Source: CAD feature listing. Evaluate the final solid. Frame: model axes, mm. A direction names the side the tool comes from. Coordinates: 2 decimals unless noted, no trailing zeros. Write each loop counter-clockwise with the first axis right and the second up, starting at its lowest first coordinate (ties: lowest second). Pieces come first, ordered by that corner, then holes. Notation, with made-up numbers: (61, 0) - (99, 0) arc R16 ccw to (99, 24) - close; hole circle Ø11 at (-11.5, -39.5). An arc over 180 degrees is marked (long way). One line per question, with ' | ' between items.
Autodesk Inventor part; units mm, degrees
ref_plane "YZ Plane" through (0, 0, 0) normal (1, 0, 0) x (0, 1, 0)
ref_plane "XZ Plane" through (0, 0, 0) normal (0, 1, 0) x (-1, 0, 0)
ref_plane "XY Plane" through (0, 0, 0) normal (0, 0, 1) x (1, 0, 0)
sketch "Sketch1" plane through (0, 0, 0) normal (0, 1, 0) x (-1, 0, 0)
  line L0 (0, 0) -> (0, -12.7)
  line L1 (0, -12.7) -> (50.8, -12.7)
  line L2 (0, 12.7) -> (50.8, 12.7)
  line L3 (50.8, -12.7) -> (50.8, 0) construction
  line L4 (50.8, 0) -> (79.375, 0) construction
  circle A0 centre (79.375, 0) radius 14.2875
  arc A1 (50.2756, -12.7) -> (50.2756, 12.7) centre (79.375, 0) ccw
  line L5 (0, 0) -> (19.05, 0) construction
  circle A2 centre (19.05, 0) radius 2.5797
  circle A3 centre (0, 0) radius 2.5797
  line L6 (0, -12.7) -> (-12.7, -12.7)
  line L7 (-12.7, -12.7) -> (-12.7, 12.7)
  line L8 (-12.7, 12.7) -> (0, 12.7)
  line L9 (-12.7, 0) -> (0, 0) construction
  dimension "d1" = 50.8
  dimension "d2" = 28.575
  dimension "d3" = 28.575
  dimension "d4" = 63.5
  dimension "d6" = 19.05
  dimension "d7" = 5.1594
  dimension "d8" = 5.1594
  dimension "d11" = 12.7
  dimension "d14" = 12.7
extrude "Extrusion1" add sketch "Sketch1" along normal blind 3.175
properties part number "wheel tip"
Item 1: Pin query (flat end, axial travel): pin 1 Ø1 at (x, y) = (-14, 1) entering from +Z; pin 2 Ø1 at (y, z) = (1, 14) entering from +X; pin 3 Ø1.5 at (x, y) = (-70, 1) entering from -Z. Return the tip coordinate at first contact, or that it passes through.
Check sheet entries:
pin 1: z = 12.7 | pin 2: x = -50.64 | pin 3: z = -30.56
Item 2: Mould query, pull axis X, two halves, no side actions, for faces 1 (the face through (1.901, 1.565, -1.743)), 2 (the face through (12.7, 2, 0)), 3 (the face through (-16.473, 1.565, -0.113)), 4 (the face through (-19, 2, -12.7)). Classes: pulls with the +X half, pulls with the -X half, needs draft (parallel to the pull), parting line crosses it, or undercut.
Check sheet entries:
face 1: undercut | face 2: pulls with the +X half | face 3: undercut | face 4: needs draft
Item 3: Cut plane B-B on z = 0. Return loops of the section in (x, y) (1 decimal), and give its area (3 significant figures).
Check sheet entries:
outline: (-111.1, 0) - (-93.7, 0) - (-93.7, 3.2) - (-111.1, 3.2) - close; (-65.1, 0) - (-21.6, 0) - (-21.6, 3.2) - (-65.1, 3.2) - close; (-16.5, 0) - (-2.6, 0) - (-2.6, 3.2) - (-16.5, 3.2) - close; (2.6, 0) - (12.7, 0) - (12.7, 3.2) - (2.6, 3.2) - close | area: 270 mm²
Item 4: Cut plane D-D on x = -72.5. Return loops of the section in (y, z) (3 decimals).
Check sheet entries:
outline: (0, -30.997) - (3.175, -30.997) - (3.175, -12.525) - (0, -12.525) - close; (0, 12.525) - (3.175, 12.525) - (3.175, 30.997) - (0, 30.997) - close
Item 5: Ray query, line 1 along Z through (x, y) = (0, 1.85); line 2 along Z through (x, y) = (-87.5, 1); line 3 along X through (y, z) = (1.55, 13). Return the intervals inside material, ascending. Write a range as [from, to].
Check sheet entries:
line 1: [-12.7, -2.58], [2.58, 12.7] | line 2: [-30.69, -11.75], [11.75, 30.69] | line 3: [-108.34, -85.3], [-73.45, -50.41]
Item 6: Cut plane A-A on x = 0. Return loops of the section in (y, z) (3 decimals).
Check sheet entries:
outline: (0, -12.7) - (3.175, -12.7) - (3.175, -2.58) - (0, -2.58) - close; (0, 2.58) - (3.175, 2.58) - (3.175, 12.7) - (0, 12.7) - close
Item 7: Cut plane C-C on y = 1.7. State how many separate pieces and enclosed holes the cut face has, and give its area (3 significant figures).
Check sheet entries:
separate pieces: 1 | enclosed holes: 3 | area: 4,040 mm²
Item 8: Access query for faces 5 (the face through (-111.1, 1.57, 1.21)), 6 (the face through (-18, 2, 12.7)). Directions: +Z, -Z, +X, -X, +Y, -Y. A direction counts if a zero-diameter tool reaches every point of the face in a straight line with its end or side. Return the directions, or none.
Check sheet entries:
face 5: +Y, -Y | face 6: +Z, +X, +Y, -Y
